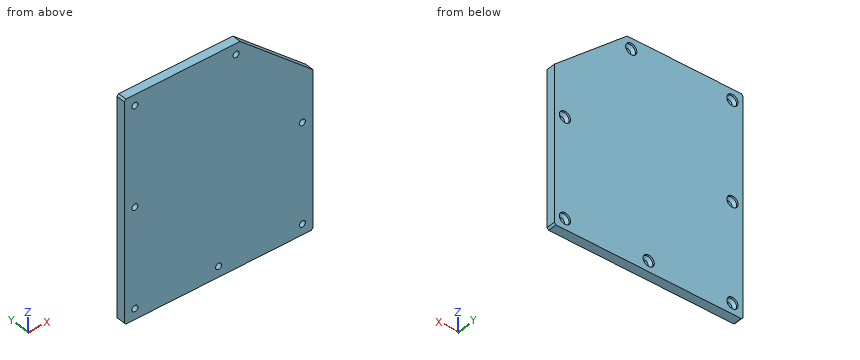
from build123d import *

# Parameters (mm, degrees)
BOSS_EXTRUDE1_DEPTH                          = 5
CSK_FOR_M3_COUNTERSUNK_FLAT_HEAD_SCR_2_COUNT = 2
CSK_FOR_M3_COUNTERSUNK_FLAT_HEAD_SCR_2_PITCH = 47
CSK_FOR_M3_COUNTERSUNK_FLAT_HEAD_SCR_3_COUNT = 2
CSK_FOR_M3_COUNTERSUNK_FLAT_HEAD_SCR_3_PITCH = 94
CSK_FOR_M3_COUNTERSUNK_FLAT_HEAD_SCR_4_COUNT = 2
CSK_FOR_M3_COUNTERSUNK_FLAT_HEAD_SCR_4_PITCH = 109.16157749
CSK_FOR_M3_COUNTERSUNK_FLAT_HEAD_SCR_5_COUNT = 2
CSK_FOR_M3_COUNTERSUNK_FLAT_HEAD_SCR_5_PITCH = 124.687328624
CSK_FOR_M3_COUNTERSUNK_FLAT_HEAD_SCR_6_COUNT = 2
CSK_FOR_M3_COUNTERSUNK_FLAT_HEAD_SCR_6_PITCH = 111
CSK_FOR_M3_COUNTERSUNK_FLAT_HEAD_SCR_7_COUNT = 2
CSK_FOR_M3_COUNTERSUNK_FLAT_HEAD_SCR_7_PITCH = 55.5


with BuildPart() as part:
    # block_perimeter → Boss-Extrude1 (new body)
    with BuildSketch(Plane(origin=(0, 0, 0), x_dir=(1, 0, 0), z_dir=(0, 1, 0))):
        Polygon((52, 60.5), (-52, 60.5), (-53, 59.5), (-53, -61.5), (-52, -62.5), (12.040578429, -62.5), (53, -26.89451804), (53, 59.5), align=None)
    extrude(amount=BOSS_EXTRUDE1_DEPTH)

    # Sketch5 → CSK for M3 Countersunk Flat Head Screw1 (revolve, cut)
    with BuildSketch(Plane(origin=(-47, 5, -54.5), x_dir=(0, 0, 1), z_dir=(1, 0, 0))):
        Polygon((0, 0), (0, 5), (1.7, 5), (1.7, 2.45), (3.15, 1), (3.15, 0), align=None)
    csk_for_m3_countersunk_flat_head_screw1 = revolve(axis=Axis((-47, 11.35, -54.5), (0, -1, 0)), mode=Mode.SUBTRACT)

    # CSK for M3 Countersunk Flat Head Scr 2: CSK for M3 Countersunk Flat Head Screw1 ×2
    with Locations(*[(i * CSK_FOR_M3_COUNTERSUNK_FLAT_HEAD_SCR_2_PITCH, 0, 0) for i in range(1, CSK_FOR_M3_COUNTERSUNK_FLAT_HEAD_SCR_2_COUNT)]):
        add(csk_for_m3_countersunk_flat_head_screw1, mode=Mode.SUBTRACT)

    # CSK for M3 Countersunk Flat Head Scr 3: CSK for M3 Countersunk Flat Head Screw1 ×2
    with Locations(*[(i * CSK_FOR_M3_COUNTERSUNK_FLAT_HEAD_SCR_3_PITCH, 0, 0) for i in range(1, CSK_FOR_M3_COUNTERSUNK_FLAT_HEAD_SCR_3_COUNT)]):
        add(csk_for_m3_countersunk_flat_head_screw1, mode=Mode.SUBTRACT)

    # CSK for M3 Countersunk Flat Head Scr 4: CSK for M3 Countersunk Flat Head Screw1 ×2
    with Locations(*[Vector(0.8611088458210153, 0, 0.508420648330493) * (i * CSK_FOR_M3_COUNTERSUNK_FLAT_HEAD_SCR_4_PITCH) for i in range(1, CSK_FOR_M3_COUNTERSUNK_FLAT_HEAD_SCR_4_COUNT)]):
        add(csk_for_m3_countersunk_flat_head_screw1, mode=Mode.SUBTRACT)

    # CSK for M3 Countersunk Flat Head Scr 5: CSK for M3 Countersunk Flat Head Screw1 ×2
    with Locations(*[Vector(0.4555175812861699, 0, 0.8902267874756397) * (i * CSK_FOR_M3_COUNTERSUNK_FLAT_HEAD_SCR_5_PITCH) for i in range(1, CSK_FOR_M3_COUNTERSUNK_FLAT_HEAD_SCR_5_COUNT)]):
        add(csk_for_m3_countersunk_flat_head_screw1, mode=Mode.SUBTRACT)

    # CSK for M3 Countersunk Flat Head Scr 6: CSK for M3 Countersunk Flat Head Screw1 ×2
    with Locations(*[(0, 0, i * CSK_FOR_M3_COUNTERSUNK_FLAT_HEAD_SCR_6_PITCH) for i in range(1, CSK_FOR_M3_COUNTERSUNK_FLAT_HEAD_SCR_6_COUNT)]):
        add(csk_for_m3_countersunk_flat_head_screw1, mode=Mode.SUBTRACT)

    # CSK for M3 Countersunk Flat Head Scr 7: CSK for M3 Countersunk Flat Head Screw1 ×2
    with Locations(*[(0, 0, i * CSK_FOR_M3_COUNTERSUNK_FLAT_HEAD_SCR_7_PITCH) for i in range(1, CSK_FOR_M3_COUNTERSUNK_FLAT_HEAD_SCR_7_COUNT)]):
        add(csk_for_m3_countersunk_flat_head_screw1, mode=Mode.SUBTRACT)


solid = part.part
Geometry check sheet. Reference: the model listing, model coordinates, mm. Round coordinates to 2 decimals unless told otherwise and drop trailing zeros. Loops run counter-clockwise (first coordinate to the right, second up) from the corner with the lowest first, then second, coordinate; pieces in that order, holes last. Notation, with made-up numbers: (19.5, 32) -> (75.5, 32) arc R35 cw to (75.5, 68) -> close; hole circle Ø6 at (67, 14.25). An arc over 180 degrees is marked (long way). Answer as a JSON object with one key per item and string values. Group by question number.
Item 1: Cross-section at A-A, the plane x = -47. Record the cut outline in (y, z), plus the area to 3 significant figures.
Item 2: Thickness scan on line 1 along Z through (x, y) = (-47, 0.6); line 2 along X through (y, z) = (1.2, 1); line 3 along Z through (x, y) = (-47, 4.4). Record the ranges inside material, lowest first.
Item 3: Depth check by flat-ended pin: pin 1 Ø5.5 at (x, z) = (9.8, 56.5) entering from +Y; pin 2 Ø5 at (x, z) = (47, 1) entering from +Y. Enter the tip coordinate at first touch or a pass-through.
Item 4: Cross-section at C-C, the plane y = 1.1. Record the cut outline in (x, z).
Item 5: Cross-section at B-B, the plane z = -54.5. Record the cut outline in (x, y).
Item 6: Cross-section at D-D, the plane z = 1. Record the cut outline in (x, y).
Determined:
{
 "1": {"outline": "(0, -60.5) -> (5, -60.5) -> (5, -57.65) -> (4, -57.65) -> (2.55, -56.2) -> (0, -56.2) -> close; (0, -52.8) -> (2.55, -52.8) -> (4, -51.35) -> (5, -51.35) -> (5, -2.15) -> (4, -2.15) -> (2.55, -0.7) -> (0, -0.7) -> close; (0, 2.7) -> (2.55, 2.7) -> (4, 4.15) -> (5, 4.15) -> (5, 53.35) -> (4, 53.35) -> (2.55, 54.8) -> (0, 54.8) -> close; (0, 58.2) -> (2.55, 58.2) -> (4, 59.65) -> (5, 59.65) -> (5, 62.5) -> (0, 62.5) -> close", "area": "549 mm²"},
 "2": {"line 1": "z = -60.5 to -56.2, -52.8 to -0.7, 2.7 to 54.8, 58.2 to 62.5", "line 2": "x = -53 to -48.7, -45.3 to 45.3, 48.7 to 53", "line 3": "z = -60.5 to -57.65, -51.35 to -2.15, 4.15 to 53.35, 59.65 to 62.5"},
 "3": {"pin 1": "stops at y = 3.6", "pin 2": "stops at y = 3.35"},
 "4": {"outline": "(-53, -59.5) -> (-52, -60.5) -> (52, -60.5) -> (53, -59.5) -> (53, 26.89) -> (12.04, 62.5) -> (-52, 62.5) -> (-53, 61.5) -> close; hole circle Ø3.4 at (-47, -54.5); hole circle Ø3.4 at (-47, 1); hole circle Ø3.4 at (-47, 56.5); hole circle Ø3.4 at (0, -54.5); hole circle Ø3.4 at (9.8, 56.5); hole circle Ø3.4 at (47, -54.5); hole circle Ø3.4 at (47, 1)"},
 "5": {"outline": "(-53, 0) -> (-48.7, 0) -> (-48.7, 2.55) -> (-50.15, 4) -> (-50.15, 5) -> (-53, 5) -> close; (-45.3, 0) -> (-1.7, 0) -> (-1.7, 2.55) -> (-3.15, 4) -> (-3.15, 5) -> (-43.85, 5) -> (-43.85, 4) -> (-45.3, 2.55) -> close; (1.7, 0) -> (45.3, 0) -> (45.3, 2.55) -> (43.85, 4) -> (43.85, 5) -> (3.15, 5) -> (3.15, 4) -> (1.7, 2.55) -> close; (48.7, 0) -> (53, 0) -> (53, 5) -> (50.15, 5) -> (50.15, 4) -> (48.7, 2.55) -> close"},
 "6": {"outline": "(-53, 0) -> (-48.7, 0) -> (-48.7, 2.55) -> (-50.15, 4) -> (-50.15, 5) -> (-53, 5) -> close; (-45.3, 0) -> (45.3, 0) -> (45.3, 2.55) -> (43.85, 4) -> (43.85, 5) -> (-43.85, 5) -> (-43.85, 4) -> (-45.3, 2.55) -> close; (48.7, 0) -> (53, 0) -> (53, 5) -> (50.15, 5) -> (50.15, 4) -> (48.7, 2.55) -> close"}
}
